```python
from build123d import *

# Parameters (mm, degrees)
SKETCH1_R           = 70
BOSS_EXTRUDE1_DEPTH = 2
CUT_EXTRUDE2_REACH  = 4
SKETCH5_R           = 16
SKETCH6_R           = 7.5
CUT_EXTRUDE3_DEPTH  = 10
SKETCH7_R           = 1
BOSS_EXTRUDE2_DEPTH = 4
FILLET1_R           = 1


with BuildPart() as part:
    # Sketch1 → Boss-Extrude1 (new body)
    with BuildSketch(Plane(origin=(0, 0, 0), x_dir=(1, 0, 0), z_dir=(0, 1, 0))):
        Circle(SKETCH1_R)
    extrude(amount=BOSS_EXTRUDE1_DEPTH)

    # Sketch5 → Cut-Extrude2 (cut, up to next)
    with BuildSketch(Plane(origin=(0, 2, 0), x_dir=(1, 0, 0), z_dir=(0, 1, 0)), mode=Mode.PRIVATE) as cut_extrude2_sk1:
        Circle(SKETCH5_R)
    cut_extrude2_tool1 = extrude(cut_extrude2_sk1.sketch, amount=-CUT_EXTRUDE2_REACH, mode=Mode.PRIVATE) & part.part
    add(cut_extrude2_tool1.solids().sort_by_distance((0, 2, 0))[0], mode=Mode.SUBTRACT)

    # Sketch6 → Cut-Extrude3 (cut)
    with BuildSketch(Plane(origin=(0, 2, 0), x_dir=(1, 0, 0), z_dir=(0, 1, 0))):
        with Locations((0, -49.88)):
            Circle(SKETCH6_R)
    extrude(amount=-CUT_EXTRUDE3_DEPTH, mode=Mode.SUBTRACT)

    # Sketch7 → Boss-Extrude2 (add)
    with BuildSketch(Plane(origin=(0, 0, 0), x_dir=(1, 0, 0), z_dir=(0, 1, 0))):
        with Locations((0, -60.88)):
            Circle(SKETCH7_R)
    extrude(amount=-BOSS_EXTRUDE2_DEPTH)

    # Fillet1
    fillet1_edges = [part.edges().sort_by_distance(p)[0] for p in [
        (-1, -4, 60.88),
    ]]
    fillet(fillet1_edges, radius=FILLET1_R)


solid = part.part
```
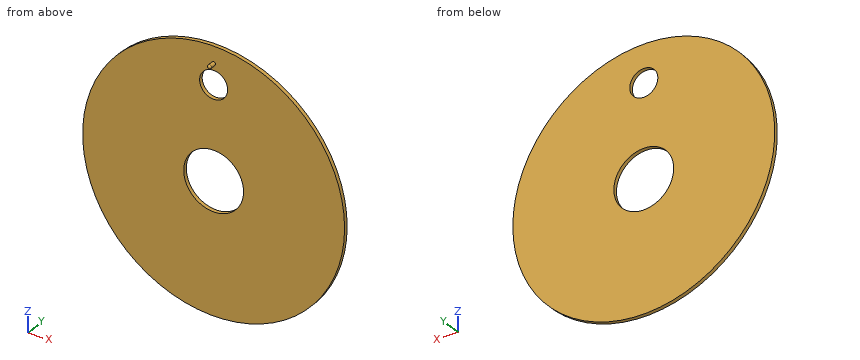
Input: part model. Units: mm. Frame: model coordinates. Coordinates: 2 decimals unless noted, no trailing zeros. Loops run counter-clockwise (first coordinate to the right, second up) from the corner with the lowest first, then second, coordinate; pieces in that order, holes last. Notation, with made-up numbers: M 79,-35 L 84,-35 A25 cw 84,-10 Z; hole C 62.5,-40 d10. An arc over 180 degrees is marked long. Use a Markdown table: item, result. Add a question column.
1) Line query: L1, parallel to Z at x = 0, y = 0.8; L2, parallel to X at y = 0.45, z = 0; L3, parallel to Y at x = 38.5, z = 28. Output: solid intervals per line, ascending. Write a range as from..to.
2) Section B-B, the plane x = -4. Return the cut outline in (y, z), plus the area to 3 significant figures.
3) Section A-A, the plane z = 0. Return the cut outline in (x, y).
4) Section D-D, the plane y = -1.4. Return the cut outline in (x, z).
5) Section C-C, the plane z = 51.5. Return the cut outline in (x, y), plus the area to 3 significant figures.
6) Pin query (flat end, axial travel): P1, Ø10, axis at x = -52, z = -6.5, coming from the -Y side; P2, Ø1, axis at y = 0, z = 30.5, coming from the +X side; P3, Ø1.5, axis at x = -26.5, y = -2.5, coming from the +Z side. Return the tip coordinate at first contact, or that it passes through.
Answer below:
| question | item | result |
|---|---|---|
| 1 | L1 | -70..-16, 16..42.38, 57.38..70 |
| 1 | L2 | -70..-16, 16..70 |
| 1 | L3 | 0..2 |
| 2 | outline | M 0,-69.89 L 2,-69.89 L 2,-15.49 L 0,-15.49 Z; M 0,15.49 L 2,15.49 L 2,43.54 L 0,43.54 Z; M 0,56.22 L 2,56.22 L 2,69.89 L 0,69.89 Z |
| 2 | area | 192 mm2 |
| 3 | outline | M -70,0 L -16,0 L -16,2 L -70,2 Z; M 16,0 L 70,0 L 70,2 L 16,2 Z |
| 4 | outline | C 0,60.88 d2 |
| 5 | outline | M -47.41,0 L -7.32,0 L -7.32,2 L -47.41,2 Z; M 7.32,0 L 47.41,0 L 47.41,2 L 7.32,2 Z |
| 5 | area | 160 mm2 |
| 6 | P1 | y = 0 |
| 6 | P2 | x = 63.25 |
| 6 | P3 | through |
